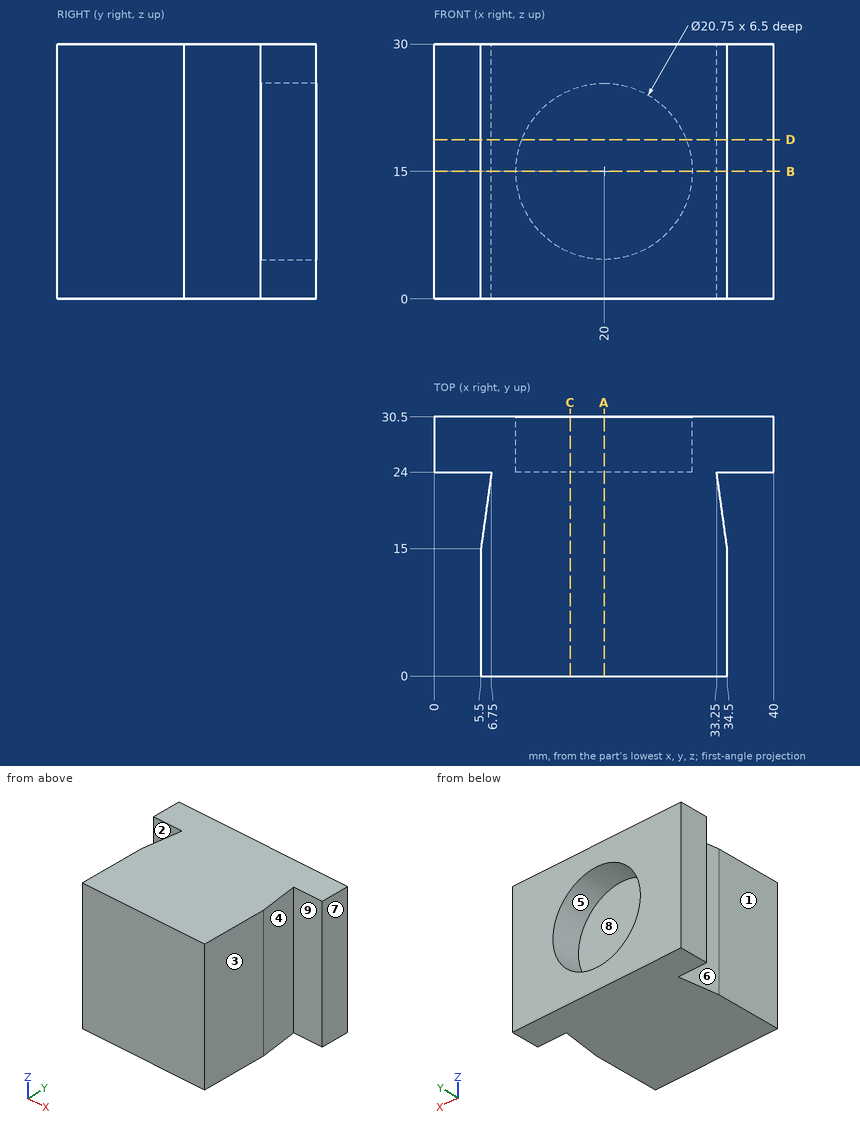
Here's the drawing with two shaded views (mm, measured from the low corner). I have some questions. A direction names the side the tool comes from. Give positions to 0.01 mm unless a question says otherwise; leave off trailing zeros. Write each loop counter-clockwise with the first axis right and the second up, starting at its lowest first coordinate (ties: lowest second). Pieces come first, ordered by that corner, then holes. Notation, with made-up numbers: (0.25, 5) - (24.25, 5) arc R22 cw to (24.25, 33) - close; hole circle Ø7 at (40.25, -29). An arc over 180 degrees is marked (long way). Write item = value, one per line. Start each with the question number.
1. For pin 1 (4.5 mm diameter, centred on y = 4, z = 10.5, fed in from +X); pin 2 (2 mm diameter, centred on x = 36, z = 12, fed in from -Y); pin 3 (3 mm diameter, centred on x = 22, y = 26, fed in from -Z); pin 4 (4.5 mm diameter, centred on y = 5.5, z = 14.5, fed in from -X), each with a flat end and sliding along its axis, tell me the tip position at first contact or that it passes through.
2. Please list where these lines run through material, in increasing order: line 1 (X direction, y = 28.25, z = 15) (3 decimals); line 2 (X direction, y = 7.5, z = 14.25); line 3 (Y direction, x = 28, z = 17.75).
3. Imagine slicing it at C-C (x = 16). Please give me the cut outline in (y, z).
4. Imagine slicing it at D-D (z = 18.75). Please give me the cut outline in (x, y), and give its area (3 significant figures).
5. Imagine slicing it at B-B (z = 15). Please give me the cut outline in (x, y) (3 decimals).
6. Imagine slicing it at A-A (x = 20). Please give me the cut outline in (y, z) (3 decimals).
7. Thinking about a two-plate mould opening in Y: for the marked faces 6, 7, 8 and 9, which applies, released by +Y, released by -Y, zero draft, split by the parting line, or undercut?
8. On a 3-axis mill with a long thin cutter (end or side, diameter ignored), from which of +Z, -Z, +X, -X, +Y, -Y can I reach the whole of each face in a straight line? I mean the marked faces 1, 2, 3, 4 and 5. Say none if no direction works.
Worked answers:
q1.pin_1 = 34.5
q1.pin_2 = 24
q1.pin_3 = 0
q1.pin_4 = 5.5
q2.line_1 = 0 to 9.625, 30.375 to 40
q2.line_2 = 5.5 to 34.5
q2.line_3 = 0 to 24
q3.outline = (0, 0) - (30.5, 0) - (30.5, 5.43) - (24, 5.43) - (24, 24.57) - (30.5, 24.57) - (30.5, 30) - (0, 30) - close
q4.outline = (0, 24) - (6.75, 24) - (5.5, 15) - (5.5, 0) - (34.5, 0) - (34.5, 15) - (33.25, 24) - (40, 24) - (40, 30.5) - (29.67, 30.5) - (29.67, 24) - (10.33, 24) - (10.33, 30.5) - (0, 30.5) - close
q4.area = 819 mm2
q5.outline = (0, 24) - (6.75, 24) - (5.5, 15) - (5.5, 0) - (34.5, 0) - (34.5, 15) - (33.25, 24) - (40, 24) - (40, 30.5) - (30.375, 30.5) - (30.375, 24) - (9.625, 24) - (9.625, 30.5) - (0, 30.5) - close
q6.outline = (0, 0) - (30.5, 0) - (30.5, 4.625) - (24, 4.625) - (24, 25.375) - (30.5, 25.375) - (30.5, 30) - (0, 30) - close
q7.face_6 = undercut
q7.face_7 = zero draft
q7.face_8 = released by +Y
q7.face_9 = undercut
q8.face_1 = +Z, -Z, -X, -Y
q8.face_2 = +Z, -Z, -X
q8.face_3 = +Z, -Z, +X, -Y
q8.face_4 = +Z, -Z, +X
q8.face_5 = +Y
